from build123d import *

# Parameters (mm, degrees)
EXTRUDE_1_DEPTH          = 12.5
CUT_EXTRUDE_1_DEPTH      = 20.532024985
CUT_EXTRUDE_1_DEPTH_BACK = 20.532024985
SKETCH_2_R               = 2
CUT_EXTRUDE_2_DEPTH      = 20.532024985
CUT_EXTRUDE_2_DEPTH_BACK = 20.532024985
CUT_EXTRUDE_START        = 12.5
SKETCH_5_W               = 16
SKETCH_5_H               = 5
CUT_EXTRUDE_4_DEPTH      = 5.5
CUT_EXTRUDE_5_DEPTH      = 2.5
CUT_EXTRUDE_5_DEPTH_BACK = 2.5
EXTRUDE_START            = 12.5
EXTRUDE_5_DEPTH          = 1.5
SKETCH_8_R               = 1
CUT_EXTRUDE_6_DEPTH      = 1.5
CUT_EXTRUDE_START_2      = 14
CUT_EXTRUDE_7_DEPTH      = 1.5


with BuildPart() as part:
    # 草图1 → 凸台-拉伸1 (new body)
    with BuildSketch(Plane(origin=(0, 0, 0), x_dir=(1, 0, 0), z_dir=(0, 1, 0))):
        Polygon((13, 5.5), (8, 5.5), (8, -5.5), (13, -5.5), (13, -7.5), (-13, -7.5), (-13, -5.5), (-8, -5.5), (-8, 5.5), (-13, 5.5), (-13, 7.5), (13, 7.5), align=None)
    extrude(amount=EXTRUDE_1_DEPTH)

    # 草图2 → 切除-拉伸1 (cut, two sides: drawn at the far end of the back side and taken through both)
    with BuildSketch(Plane.XY.offset(-CUT_EXTRUDE_1_DEPTH_BACK)):
        with Locations((0, 3.5)):
            Circle(SKETCH_2_R)
    extrude(amount=CUT_EXTRUDE_1_DEPTH + CUT_EXTRUDE_1_DEPTH_BACK, mode=Mode.SUBTRACT)

    # 草图3 → 切除-拉伸2 (cut, two sides: drawn at the far end of the back side and taken through both)
    with BuildSketch(Plane.XY.offset(-CUT_EXTRUDE_2_DEPTH_BACK)):
        with BuildLine():
            Line((-10.5, 11), (-2, 11))
            ThreePointArc((-2, 11), (-1, 10), (-2, 9))
            Line((-2, 9), (-10.5, 9))
            ThreePointArc((-10.5, 9), (-11.5, 10), (-10.5, 11))
        make_face()
        with BuildLine():
            Line((2, 9), (10.5, 9))
            ThreePointArc((10.5, 9), (11.5, 10), (10.5, 11))
            Line((10.5, 11), (2, 11))
            ThreePointArc((2, 11), (1, 10), (2, 9))
        make_face()
    extrude(amount=CUT_EXTRUDE_2_DEPTH + CUT_EXTRUDE_2_DEPTH_BACK, mode=Mode.SUBTRACT)

    # 草图5 → 切除-拉伸4 (cut)
    with BuildSketch(Plane(origin=(0, 0, 0), x_dir=(1, 0, 0), z_dir=(0, 1, 0)).offset(CUT_EXTRUDE_START)):
        Rectangle(SKETCH_5_W, SKETCH_5_H)
    extrude(amount=-CUT_EXTRUDE_4_DEPTH, mode=Mode.SUBTRACT)

    # 草图6 → 切除-拉伸5 (cut, two sides: drawn at the far end of the back side and taken through both)
    with BuildSketch(Plane.XY.offset(-CUT_EXTRUDE_5_DEPTH_BACK)):
        with BuildLine():
            Line((8, 7), (0, 7))
            ThreePointArc((0, 7), (4.949747468, 4.949747468), (7, 0))
            Line((7, 0), (8, 0))
            Line((8, 0), (8, 7))
        make_face()
        with BuildLine():
            Line((-8, 7), (-8, 0))
            Line((-8, 0), (-7, 0))
            ThreePointArc((-7, 0), (-4.949747468, 4.949747468), (0, 7))
            Line((0, 7), (-8, 7))
        make_face()
    extrude(amount=CUT_EXTRUDE_5_DEPTH + CUT_EXTRUDE_5_DEPTH_BACK, mode=Mode.SUBTRACT)

    # 草图7 → 凸台-拉伸5 (add)
    with BuildSketch(Plane(origin=(0, 0, 0), x_dir=(1, 0, 0), z_dir=(0, 1, 0)).offset(EXTRUDE_START)):
        with BuildLine():
            Line((17.82554347, 2.5), (15.07554347, 2.5))
            Line((15.07554347, 2.5), (15.07554347, -2.5))
            Line((15.07554347, -2.5), (17.82554347, -2.5))
            ThreePointArc((17.82554347, -2.5), (0, -18), (-17.82554347, -2.5))
            Line((-17.82554347, -2.5), (-15.07554347, -2.5))
            Line((-15.07554347, -2.5), (-15.07554347, 2.5))
            Line((-15.07554347, 2.5), (-17.82554347, 2.5))
            ThreePointArc((-17.82554347, 2.5), (0, 18), (17.82554347, 2.5))
        make_face()
    extrude(amount=EXTRUDE_5_DEPTH)

    # 草图8 → 切除-拉伸6 (cut)
    with BuildSketch(Plane(origin=(0, 0, 0), x_dir=(1, 0, 0), z_dir=(0, 1, 0)).offset(CUT_EXTRUDE_START)):
        with Locations(Location((0, 12.5, 0), (0, 0, 270))):
            Circle(SKETCH_8_R)
        with Locations(Location((0, -12.5, 0), (0, 0, 270))):
            Circle(SKETCH_8_R)
    extrude(amount=CUT_EXTRUDE_6_DEPTH, mode=Mode.SUBTRACT)

    # 草图9 → 切除-拉伸7 (cut)
    with BuildSketch(Plane(origin=(0, 0, 0), x_dir=(1, 0, 0), z_dir=(0, 1, 0)).offset(CUT_EXTRUDE_START_2)):
        with BuildLine():
            Line((-12.02081528, 10.606601718), (-13.435028843, 12.02081528))
            ThreePointArc((-13.435028843, 12.02081528), (-13.435028843, 13.435028843), (-12.02081528, 13.435028843))
            Line((-12.02081528, 13.435028843), (-10.606601718, 12.02081528))
            ThreePointArc((-10.606601718, 12.02081528), (-10.606601718, 10.606601718), (-12.02081528, 10.606601718))
        make_face()
        with BuildLine():
            Line((10.606601718, -12.02081528), (12.02081528, -13.435028843))
            ThreePointArc((12.02081528, -13.435028843), (13.435028843, -13.435028843), (13.435028843, -12.02081528))
            Line((13.435028843, -12.02081528), (12.02081528, -10.606601718))
            ThreePointArc((12.02081528, -10.606601718), (10.606601718, -10.606601718), (10.606601718, -12.02081528))
        make_face()
        with BuildLine():
            Line((-12.02081528, -10.606601718), (-13.435028843, -12.02081528))
            ThreePointArc((-13.435028843, -12.02081528), (-13.435028843, -13.435028843), (-12.02081528, -13.435028843))
            Line((-12.02081528, -13.435028843), (-10.606601718, -12.02081528))
            ThreePointArc((-10.606601718, -12.02081528), (-10.606601718, -10.606601718), (-12.02081528, -10.606601718))
        make_face()
        with BuildLine():
            Line((10.606601718, 12.02081528), (12.02081528, 13.435028843))
            ThreePointArc((12.02081528, 13.435028843), (13.435028843, 13.435028843), (13.435028843, 12.02081528))
            Line((13.435028843, 12.02081528), (12.02081528, 10.606601718))
            ThreePointArc((12.02081528, 10.606601718), (10.606601718, 10.606601718), (10.606601718, 12.02081528))
        make_face()
    extrude(amount=-CUT_EXTRUDE_7_DEPTH, mode=Mode.SUBTRACT)


solid = part.part
Model file for the job. Use its own axes, mm. A direction names the side the tool comes from. Coordinates: 2 decimals unless noted, no trailing zeros. Order: outer loops, then holes, each group sorted by start corner. A loop starts at its lowest first (then second) coordinate and runs counter-clockwise, first axis right, second up. Notation, with made-up numbers: M 42.25,6 L 75.25,6 A10 cw 75.25,19 Z; hole C 51.5,-16.5 d5. An arc over 180 degrees is marked long. Return JSON: item names as keys, results as strings.
1. Saw through at C-C (y = 4.75). Give the cut face in (x, z).
Ans:
{"outline": "M -13,-7.5 L -1.56,-7.5 L -1.56,7.5 L -13,7.5 L -13,5.5 L -8,5.5 L -8,2.5 L -5.14,2.5 L -5.14,-2.5 L -8,-2.5 L -8,-5.5 L -13,-5.5 Z; M 1.56,-7.5 L 13,-7.5 L 13,-5.5 L 8,-5.5 L 8,-2.5 L 5.14,-2.5 L 5.14,2.5 L 8,2.5 L 8,5.5 L 13,5.5 L 13,7.5 L 1.56,7.5 Z"}
2. Tool access for faces 4 (the face through (16, 13, -2.5)), 5 (the face through (-12.708, 13.26, 11.294)), 6 (the face through (10, 6, 5.5)), 7 (the face through (0, 6, -7.5)), 8 (the face through (-16, 13, 2.5)): list every direction of +Z, -Z, +X, -X, +Y, -Y with a clear straight run to the whole face (end or side of a thin tool).
Ans:
{"face 4": "+X, +Y, -Y", "face 5": "+Z, +Y, -Y", "face 6": "+X, -Y", "face 7": "-Z, +X, -X, -Y", "face 8": "-X, +Y, -Y"}
3. Saw through at A-A (y = 10). Give the cut face in (x, z), and give its area (3 significant figures).
Ans:
{"outline": "M -13,-7.5 L -11.5,-7.5 L -11.5,-5.5 L -13,-5.5 Z; M -13,5.5 L -11.5,5.5 L -11.5,7.5 L -13,7.5 Z; M -1,-7.5 L 1,-7.5 L 1,-2.5 L -1,-2.5 Z; M -1,2.5 L 1,2.5 L 1,7.5 L -1,7.5 Z; M 11.5,-7.5 L 13,-7.5 L 13,-5.5 L 11.5,-5.5 Z; M 11.5,5.5 L 13,5.5 L 13,7.5 L 11.5,7.5 Z", "area": "32.0 mm^2"}
4. Saw through at B-B (x = -4). Give the cut face in (y, z), and give its area (3 significant figures).
Ans:
{"outline": "M 0,-7.5 L 9,-7.5 L 9,-2.5 L 5.74,-2.5 L 5.74,2.5 L 9,2.5 L 9,7.5 L 0,7.5 Z; M 11,-7.5 L 12.5,-7.5 L 12.5,-17.55 L 14,-17.55 L 14,17.55 L 12.5,17.55 L 12.5,7.5 L 11,7.5 L 11,2.5 L 12.5,2.5 L 12.5,-2.5 L 11,-2.5 Z", "area": "186 mm^2"}
5. Saw through at D-D (x = 7.5). Give the cut face in (y, z).
Ans:
{"outline": "M 0,-7.5 L 9,-7.5 L 9,-2.5 L 0,-2.5 Z; M 0,2.5 L 9,2.5 L 9,7.5 L 0,7.5 Z; M 11,-7.5 L 12.5,-7.5 L 12.5,-16.36 L 14,-16.36 L 14,16.36 L 12.5,16.36 L 12.5,7.5 L 11,7.5 L 11,2.5 L 12.5,2.5 L 12.5,-2.5 L 11,-2.5 Z"}
6. Pull direction Z, two halves, no side cores. Call faces 1 (the face through (11.5, 10, 6.5)), 2 (the face through (12.728, 13.26, -11.314)), 3 (the face through (-8, 12, -4)): +Z half, -Z half, draft (parallel to the pull), parting line (faces both ways), or undercut.
Ans:
{"face 1": "draft", "face 2": "-Z half", "face 3": "undercut"}
7. Drill centre lines: probe 1 along Y at (x, z) = (0, -0.75); probe 2 along Z at (x, y) = (9, 3.5); probe 3 along X at (y, z) = (3.5, -3.5). Where is each one in solid material? Low to high.
Ans:
{"probe 1": "0 to 1.5, 5.5 to 7, 12.5 to 14", "probe 2": "-7.5 to -5.5, 5.5 to 7.5", "probe 3": "-8 to -2, 2 to 8"}
8. Flat gauge pins, fed straight in: pin 1 (2.5 mm diameter, centred on x = 0, z = -12.5, fed in from +Y); pin 2 (2 mm diameter, centred on x = 8, y = 6.5, fed in from -Z); pin 3 (2.5 mm diameter, centred on y = 6, z = -4, fed in from +X); pin 4 (1.5 mm diameter, centred on x = 14, z = -3.5, fed in from -Y). Where does each tip first touch, or does it go through?
Ans:
{"pin 1": "y = 14", "pin 2": "z = -7.5", "pin 3": "x = 8", "pin 4": "y = 12.5"}
